Can you work these out from the model? Positions are in its coordinate system, mm. A direction names the side the tool comes from. Coordinates: 2 decimals unless noted, no trailing zeros. Loops run counter-clockwise (first coordinate to the right, second up) from the corner with the lowest first, then second, coordinate; pieces in that order, holes last.
Autodesk Inventor part; units mm, degrees
ref_plane "YZ Plane" through (0, 0, 0) normal (1, 0, 0) x (0, 1, 0)
ref_plane "XZ Plane" through (0, 0, 0) normal (0, 1, 0) x (-1, 0, 0)
ref_plane "XY Plane" through (0, 0, 0) normal (0, 0, 1) x (1, 0, 0)
ref_plane "作業平面1" through (0, 0, 0) normal (0, 0, 1) x (1, 0, 0)
sketch "スケッチ1" plane through (0, 0, 0) normal (0, 0, 1) x (1, 0, 0)
  line L0 (5.5, -11.5) -> (-5.5, -11.5)
  line L1 (5.5, 11.5) -> (5.5, -11.5)
  line L2 (-5.5, 11.5) -> (5.5, 11.5)
  line L3 (-5.5, -11.5) -> (-5.5, 11.5)
  line L4 (2, 11.5) -> (-2, 11.5)
  line L5 (-2, 11.5) -> (-2, 15)
  line L6 (-2, 15) -> (2, 15)
  line L7 (2, 15) -> (2, 11.5)
  line L8 (2, -11.5) -> (-2, -11.5)
  line L9 (-2, -11.5) -> (-2, -15)
  line L10 (-2, -15) -> (2, -15)
  line L11 (2, -15) -> (2, -11.5)
  line L12 (0, -21) -> (0, 21)
  circle A0 centre (0, 13.25) radius 1.15
  circle A1 centre (0, -13.25) radius 1.15
  line L13 (2, 13.25) -> (-2, 13.25) construction
  line L14 (2, -13.25) -> (-2, -13.25) construction
  point P0 (0, 0)
  point P1 (0, 15)
  dimension "d0" = 3.5
  dimension "d1" = 4
  dimension "d2" = 2.3
extrude "押し出し1" add sketch "スケッチ1" along normal blind 1.6 contours L0 L12 L2 L1 | L11 L10 L12 A1 L0 | L12 A1 L10 L9 L0 | L0 L3 L2 L12 | L2 L12 A0 L6 L7 | L2 L5 L6 L12 A0
properties part number "Segment_PCB"
(1) I want a section at A-A on y = -13.25. Write out the boundary of the cut face in (x, z).
Check values:
outline: (-2, 0) - (-1.15, 0) - (-1.15, 1.6) - (-2, 1.6) - close; (1.15, 0) - (2, 0) - (2, 1.6) - (1.15, 1.6) - close
(2) I'm going to push flat-ended pins straight in: pin 1 (0.8 mm diameter, centred on x = 4.5, z = 0.5, fed in from +Y); pin 2 (2.5 mm diameter, centred on x = 0, y = -13.25, fed in from +Z); pin 3 (1.4 mm diameter, centred on x = 0, y = 13.25, fed in from -Z); pin 4 (0.5 mm diameter, centred on y = 13, z = 1, fed in from +X). Where does each tip first touch, or does it pass through?
Check values:
pin 1: stops at y = 11.5
pin 2: stops at z = 1.6
pin 3: passes through
pin 4: stops at x = 2
(3) I want a section at C-C on x = 0.5. Write out the boundary of the cut face in (y, z).
Check values:
outline: (-15, 0) - (-14.29, 0) - (-14.29, 1.6) - (-15, 1.6) - close; (-12.21, 0) - (12.21, 0) - (12.21, 1.6) - (-12.21, 1.6) - close; (14.29, 0) - (15, 0) - (15, 1.6) - (14.29, 1.6) - close
(4) If I drill on probe 1 along Y at (x, z) = (0, 0.75); probe 2 along X at (y, z) = (-13.25, 1); probe 3 along Y at (x, z) = (-2.5, 0.8), over which ranges is the centre line in solid material (lowest first)?
Check values:
probe 1: y = -15 to -14.4, -12.1 to 12.1, 14.4 to 15
probe 2: x = -2 to -1.15, 1.15 to 2
probe 3: y = -11.5 to 11.5
(5) If we mould it in two halves opening along X, with no side actions, what happens to faces 1 (the flat face through (5.5, 0, 1)), 2 (the flat face through (-5.5, 0, 1)), 3 (the cylindrical face through (0.53, -12.23, 0.79))? For each: released by +X, released by -X, zero draft, split by the parting line, or undercut.
Check values:
face 1: released by +X
face 2: released by -X
face 3: undercut
(6) Which directions (+Z, -Z, +X, -X, +Y, -Y) give clear straight access to the entire face, cutting with the end or side of a thin tool? Please do faces 4 (the flat face through (2, -13, 1)), 5 (the flat face through (-4, 11.5, 1)), 6 (the flat face through (4, 11.5, 1)), 7 (the flat face through (-2, -13, 1)), 8 (the flat face through (0, -15, 1)).
Check values:
face 4: +Z, -Z, +X, -Y
face 5: +Z, -Z, -X, +Y
face 6: +Z, -Z, +X, +Y
face 7: +Z, -Z, -X, -Y
face 8: +Z, -Z, +X, -X, -Y
(7) I want a section at B-B on z = 0.75. Write out the boundary of the cut face in (x, y).
Check values:
outline: (-5.5, -11.5) - (-2, -11.5) - (-2, -15) - (2, -15) - (2, -11.5) - (5.5, -11.5) - (5.5, 11.5) - (2, 11.5) - (2, 15) - (-2, 15) - (-2, 11.5) - (-5.5, 11.5) - close; hole circle Ø2.3 at (0, -13.25); hole circle Ø2.3 at (0, 13.25)
